```python
from build123d import *

# Parameters (mm, degrees)
SKETCH1_W             = 20.32
SKETCH1_H             = 40.64
EXTRUDE1_DEPTH        = 25.4
SKETCH2_W             = 20.32
SKETCH2_H             = 40.64
EXTRUDE2_DEPTH        = 2.38125
SKETCH3_W             = 20.32
SKETCH3_H             = 40.64
EXTRUDE3_DEPTH        = 4.445
EXTRUDE4_DEPTH        = 2.38125
SKETCH5_R             = 7.62
EXTRUDE5_DEPTH        = 3.4925
CHAMFER1_SIZE         = 2.54
CHAMFER1_SIZE2        = 1.466469684
EXTRUDE6_DEPTH        = 0.635
SKETCH8_R             = 2.778125
EXTRUDE7_DEPTH        = 3.175
CHAMFER2_SIZE         = 2.54
CHAMFER2_SIZE2        = 1.466469684
CHAMFER2_PART_2_SIZE  = 2.54
CHAMFER2_PART_2_SIZE2 = 1.466469684
FILLET1_R             = 1.016
FILLET2_R             = 1.524
SKETCH9_W             = 6.35
SKETCH9_H             = 2.54
EXTRUDE8_DEPTH        = 2.38125
SKETCH10_W            = 5.08
SKETCH10_H            = 1.27
CUT_EXTRUDE1_DEPTH    = 2.38125


with BuildPart() as part:
    # Sketch1 → Extrude1 (new body)
    with BuildSketch(Plane(origin=(0, 0, 0), x_dir=(1, 0, 0), z_dir=(0, 1, 0))):
        with Locations((0, -10.16)):
            Rectangle(SKETCH1_W, SKETCH1_H)
    extrude(amount=EXTRUDE1_DEPTH)

    # Sketch2 → Extrude2 (add)
    with BuildSketch(Plane(origin=(0, 25.4, 0), x_dir=(-1, 0, 0), z_dir=(0, 1, 0))):
        with Locations((0, 10.16)):
            Rectangle(SKETCH2_W, SKETCH2_H)
        with BuildLine():
            ThreePointArc((6.731, -15.51418631), (5.08, -11.7094), (3.429, -15.51418631))
            Line((3.429, -15.51418631), (3.429, -16.4846))
            Line((3.429, -16.4846), (-3.429, -16.4846))
            Line((-3.429, -16.4846), (-3.429, -15.51418631))
            ThreePointArc((-3.429, -15.51418631), (-5.08, -11.7094), (-6.731, -15.51418631))
            Line((-6.731, -15.51418631), (-6.731, -16.4846))
            Line((-6.731, -16.4846), (-10.16, -16.4846))
            Line((-10.16, -16.4846), (-10.16, -10.16))
            Line((-10.16, -10.16), (10.16, -10.16))
            Line((10.16, -10.16), (10.16, -16.4846))
            Line((10.16, -16.4846), (6.731, -16.4846))
            Line((6.731, -16.4846), (6.731, -15.51418631))
        make_face()
        with BuildLine():
            ThreePointArc((-6.731, 35.83418631), (-5.08, 32.0294), (-3.429, 35.83418631))
            Line((-3.429, 35.83418631), (-3.429, 36.8046))
            Line((-3.429, 36.8046), (3.429, 36.8046))
            Line((3.429, 36.8046), (3.429, 35.83418631))
            ThreePointArc((3.429, 35.83418631), (5.08, 32.0294), (6.731, 35.83418631))
            Line((6.731, 35.83418631), (6.731, 36.8046))
            Line((6.731, 36.8046), (10.16, 36.8046))
            Line((10.16, 36.8046), (10.16, 30.48))
            Line((10.16, 30.48), (-10.16, 30.48))
            Line((-10.16, 30.48), (-10.16, 36.8046))
            Line((-10.16, 36.8046), (-6.731, 36.8046))
            Line((-6.731, 36.8046), (-6.731, 35.83418631))
        make_face()
    extrude(amount=EXTRUDE2_DEPTH)

    # Sketch3 → Extrude3 (add)
    with BuildSketch(Plane(origin=(0, 27.78125, 0), x_dir=(-1, 0, 0), z_dir=(0, 1, 0))):
        with Locations((0, 10.16)):
            Rectangle(SKETCH3_W, SKETCH3_H)
    extrude(amount=EXTRUDE3_DEPTH)

    # Sketch4 → Extrude4 (add)
    with BuildSketch(Plane(origin=(0, 32.22625, 0), x_dir=(-1, 0, 0), z_dir=(0, 1, 0))):
        with BuildLine():
            Line((9.652, 2.228840954), (9.652, 24.13))
            Line((9.652, 24.13), (4.655896906, 24.13))
            ThreePointArc((4.655896906, 24.13), (0, 27.178), (-4.655896906, 24.13))
            Line((-4.655896906, 24.13), (-9.652, 24.13))
            Line((-9.652, 24.13), (-9.652, 2.228840954))
            ThreePointArc((-9.652, 2.228840954), (0, -9.906), (9.652, 2.228840954))
        make_face()
    extrude(amount=EXTRUDE4_DEPTH)

    # Sketch5 → Extrude5 (add)
    with BuildSketch(Plane(origin=(0, 34.6075, 0), x_dir=(-1, 0, 0), z_dir=(0, 1, 0))):
        Circle(SKETCH5_R)
    extrude(amount=EXTRUDE5_DEPTH)

    # Chamfer1
    chamfer1_edges = [part.edges().sort_by_distance(p)[0] for p in [
        (7.62, 38.1, 0),
    ]]
    chamfer1_side = [part.faces().sort_by_distance(p)[0] for p in [
        (0, 38.1, 0),
    ]]
    chamfer(chamfer1_edges, length=CHAMFER1_SIZE, length2=CHAMFER1_SIZE2, reference=chamfer1_side[0])

    # Sketch7 → Extrude6 (add, symmetric)
    with BuildSketch(Plane(origin=(0, 0, 0), x_dir=(0, 0, -1), z_dir=(1, 0, 0))):
        Polygon((15.494, 27.78125), (12.954, 29.55925), (10.16, 29.55925), (10.16, 27.78125), align=None)
    extrude6 = extrude(amount=EXTRUDE6_DEPTH, both=True)

    # Mirror1: Extrude6 across plane
    add(extrude6.mirror(Plane(origin=(0, 0, 10.16), x_dir=(1, 0, 0), z_dir=(0, 0, -1))))

    # Sketch8 → Extrude7 (add)
    with BuildSketch(Plane(origin=(0, 38.1, 0), x_dir=(-1, 0, 0), z_dir=(0, 1, 0))):
        Circle(SKETCH8_R)
    extrude(amount=EXTRUDE7_DEPTH)

    # Chamfer2
    chamfer2_edges = [part.edges().sort_by_distance(p)[0] for p in [
        (0, 0, -10.16),
    ]]
    chamfer2_side = [part.faces().sort_by_distance(p)[0] for p in [
        (0, 12.7, -10.16),
    ]]
    chamfer(chamfer2_edges, length=CHAMFER2_SIZE, length2=CHAMFER2_SIZE2, reference=chamfer2_side[0])

    # Chamfer2 part 2
    chamfer2_part_2_edges = [part.edges().sort_by_distance(p)[0] for p in [
        (0, 0, 30.48),
    ]]
    chamfer2_part_2_side = [part.faces().sort_by_distance(p)[0] for p in [
        (0, 12.7, 30.48),
    ]]
    chamfer(chamfer2_part_2_edges, length=CHAMFER2_PART_2_SIZE, length2=CHAMFER2_PART_2_SIZE2, reference=chamfer2_part_2_side[0])

    # Fillet1
    fillet1_edges = [part.edges().sort_by_distance(p)[0] for p in [
        (-10.16, 30.00375, -10.16),
        (10.16, 30.00375, -10.16),
        (10.16, 30.00375, 30.48),
        (10.16, 0, 10.16),
        (10.16, 1.27, -9.426765158),
        (10.16, 13.97, -10.16),
        (0, 0, -8.693530316),
        (0, 2.54, -10.16),
        (-10.16, 13.97, -10.16),
        (-10.16, 1.27, -9.426765158),
        (10.16, 13.97, 30.48),
        (10.16, 1.27, 29.746765158),
        (0, 2.54, 30.48),
        (-10.16, 0, 10.16),
        (0, 0, 29.013530316),
        (-10.16, 1.27, 29.746765158),
        (-10.16, 13.97, 30.48),
        (-10.16, 30.00375, 30.48),
    ]]
    fillet(fillet1_edges, radius=FILLET1_R)

    # Fillet2
    fillet2_edges = [part.edges().sort_by_distance(p)[0] for p in [
        (-10.16, 26.590625, 36.8046),
        (10.16, 26.590625, 36.8046),
        (-10.16, 26.590625, -16.4846),
        (10.16, 26.590625, -16.4846),
    ]]
    fillet(fillet2_edges, radius=FILLET2_R)

    # Sketch9 → Extrude8 (add)
    with BuildSketch(Plane(origin=(0, 0, -10.16), x_dir=(-1, 0, 0), z_dir=(0, 0, -1))):
        with Locations((0, 4.318)):
            Rectangle(SKETCH9_W, SKETCH9_H)
    extrude(amount=EXTRUDE8_DEPTH)

    # Sketch10 → Cut-Extrude1 (cut)
    with BuildSketch(Plane(origin=(0, 0, -12.54125), x_dir=(-1, 0, 0), z_dir=(0, 0, -1))):
        with Locations((0, 4.318)):
            Rectangle(SKETCH10_W, SKETCH10_H)
    extrude(amount=-CUT_EXTRUDE1_DEPTH, mode=Mode.SUBTRACT)


solid = part.part
```
Model file for the job. Use its own axes, mm. A direction names the side the tool comes from. Coordinates: 2 decimals unless noted, no trailing zeros. Order: outer loops, then holes, each group sorted by start corner. A loop starts at its lowest first (then second) coordinate and runs counter-clockwise, first axis right, second up. Notation, with made-up numbers: M 68.25,34.5 L 88.25,34.5 A26 ccw 88.25,50.5 Z; hole C 61,40.25 d8. An arc over 180 degrees is marked long. Answer as CSV lines item,"result".
(1) Band-saw the part on B-B, the plane y = 31.5. List the corners of the cut face in (x, z).
Geometry says:
outline,"M -10.16,-9.14 A1.02 ccw -9.14,-10.16 L 9.14,-10.16 A1.02 ccw 10.16,-9.14 L 10.16,29.46 A1.02 ccw 9.14,30.48 L -9.14,30.48 A1.02 ccw -10.16,29.46 Z"
(2) 3-axis set-ups, long thin cutter, end or side, ignore diameter. For faces 5 (the flat face through (0.635, 29, -12)), 6 (the flat face through (0.635, 29, 33)), 7 (the flat face through (0, 29.559, -12)), 8 (the flat face through (-0.635, 29, 33)): which of +Z, -Z, +X, -X, +Y, -Y reach the whole face in a straight line?
Geometry says:
face 5,"-Z, +X, +Y"
face 6,"+Z, +X, +Y"
face 7,"-Z, +X, -X, +Y"
face 8,"+Z, -X, +Y"
(3) Band-saw the part on C-C, the plane z = -13.97. List the corners of the cut face in (x, y) (3 decimals), then the cut area to 3 significant figures.
Geometry says:
outline,"M -10.16,25.4 L -7.341,25.4 L -7.341,27.781 L -10.16,27.781 Z; M -2.819,25.4 L 2.819,25.4 L 2.819,27.781 L 0.635,27.781 L 0.635,28.848 L -0.635,28.848 L -0.635,27.781 L -2.819,27.781 Z; M 7.341,25.4 L 10.16,25.4 L 10.16,27.781 L 7.341,27.781 Z"
area,"28.2 mm2"
(4) Flat gauge pins, fed straight in: pin 1 (9 mm diameter, centred on x = 4.5, y = 15.5, fed in from -Z); pin 2 (0.5 mm diameter, centred on y = 29, z = 33.5, fed in from +X) (3 decimals); pin 3 (2.5 mm diameter, centred on x = 0.5, z = -11, fed in from +Y); pin 4 (12 mm diameter, centred on x = 1, y = 21.5, fed in from +Z). Where does each tip first touch, or does it go through?
Geometry says:
pin 1,"stops at z = -10.16"
pin 2,"stops at x = 0.635"
pin 3,"stops at y = 34.61"
pin 4,"stops at z = 36.8"
(5) Wall check: line 1 along X through (y, z) = (26.65, 34.29); line 2 along Y through (x, z) = (2.5, 24); line 3 along Y through (x, z) = (-3.75, 31). Give the ranges that are in metal, low to high.
Geometry says:
line 1,"x = -10.16 to -7.34, -2.82 to 2.82, 7.34 to 10.16"
line 2,"y = 0 to 34.61"
line 3,"y = 25.4 to 27.78"
(6) Pull direction X, two halves, no side cores. Call faces 1 (the cylindrical face through (-5.01, 26.57, 32.03)), 2 (the flat face through (10.16, 16, 11)), 3 (the flat face through (-10.16, 16, 10)), 4 (the flat face through (0.01, 28.66, -14.24)): +X half, -X half, draft (parallel to the pull), parting line (faces both ways), or undercut.
Geometry says:
face 1,"undercut"
face 2,"+X half"
face 3,"-X half"
face 4,"draft"
(7) Band-saw the part on A-A, the plane z = 9. List the corners of the cut face in (x, y), then the cut area to 3 significant figures.
Geometry says:
outline,"M -10.16,1.02 A1.02 ccw -9.14,0 L 9.14,0 A1.02 ccw 10.16,1.02 L 10.16,32.23 L 9.65,32.23 L 9.65,34.61 L -9.65,34.61 L -9.65,32.23 L -10.16,32.23 Z"
area,"700 mm2"
